Autodesk Inventor part; units mm, degrees
ref_plane "YZ Plane" through (0, 0, 0) normal (1, 0, 0) x (0, 1, 0)
ref_plane "XZ Plane" through (0, 0, 0) normal (0, 1, 0) x (-1, 0, 0)
ref_plane "XY Plane" through (0, 0, 0) normal (0, 0, 1) x (1, 0, 0)
sketch "Sketch1" plane through (0, 0, 0) normal (0, 0, 1) x (1, 0, 0)
  circle A0 centre (0, 0) radius 1.5875
  dimension "d0" = 3.175
extrude "Extrusion1" add sketch "Sketch1" along normal mid plane 33.0149
sketch "Sketch2" plane through (0, 0, 16.5075) normal (0, 0, 1) x (1, 0, 0)
  circle A0 centre (0, 0) radius 1.1913
  dimension "d3" = 2.3825
extrude "Extrusion2" add sketch "Sketch2" along normal blind 0.381
sketch "Sketch3" plane through (0, 0, 16.8885) normal (0, 0, 1) x (1, 0, 0)
  circle A0 centre (0, 0) radius 1.5875
  dimension "d6" = 3.175
extrude "Extrusion3" add sketch "Sketch3" along normal blind 1.27
chamfer "Chamfer1" distance 0.381 angle 45 1 edges at (-1.5875, 0, 18.1585)
mirror "Mirror1" about plane through (0, 0, 0) normal (0, 0, 1) of "Extrusion3", "Extrusion2", "Chamfer1"
scale "Scale1" factors (10, 10, 10) then translate (0, 0, 0) bodies 1
properties part number "Front Upper Hinge Pin"
Work out the finished part from the listing and answer in its coordinate system (mm). A direction names the side the tool comes from. Round coordinates to 2 decimals unless told otherwise and drop trailing zeros. Write each loop counter-clockwise with the first axis right and the second up, starting at its lowest first coordinate (ties: lowest second). Pieces come first, ordered by that corner, then holes. Notation, with made-up numbers: (57.25, 36.5) - (95.25, 36.5) arc R3 ccw to (95.25, 40.5) - close; hole circle Ø4 at (30, -18). An arc over 180 degrees is marked (long way). Answer in a Markdown table with one row per item. Add a question column.
1. The mould has two halves that part along Z. Classify faces 1 (the flat face through (2, 12, 165.074)), 2 (the flat face through (0, 0, -181.585)), 3 (the cylindrical face through (-3.441, -15.497, 2.311)): +Z half, -Z half, draft (parallel to the pull), parting line (faces both ways), or undercut.
2. For faces 4 (the flat face through (0, 0, 181.585)), 5 (the cylindrical face through (5.497, 10.569, 166.953)), determine the directions among +Z, -Z, +X, -X, +Y, -Y from which every point of the face is accessible in a straight line to the end or side of a thin tool.
3. Find the intervals of material crossed by line 1 along Z through (x, y) = (-13, 5) (1 decimal); line 2 along Z through (x, y) = (-5, 11.5) (1 decimal); line 3 along X through (y, z) = (-10.5, 4), in increasing order. Write a range as from..to.
4. Given pin 1 (3 mm diameter, centred on x = 8.5, z = 67.5, fed in from -Y); pin 2 (6 mm diameter, centred on y = 8, z = 23, fed in from +X); pin 3 (1.5 mm diameter, centred on y = -9, z = -81.5, fed in from +X), each flat-ended and moving along its own axis, determine where each tip first touches the part or whether it passes through.
5. A cutting plane is placed at A-A, the plane z = -25.5. Determine the outline of the cut face in (x, y) (3 decimals), and give its area (3 significant figures).
Worked out:
| question | item | result |
|---|---|---|
| 1 | face 1 | undercut |
| 1 | face 2 | -Z half |
| 1 | face 3 | draft |
| 2 | face 4 | +Z, +X, -X, +Y, -Y |
| 2 | face 5 | none |
| 3 | line 1 | -179.7..-168.9, -165.1..165.1, 168.9..179.7 |
| 3 | line 2 | -181.1..-168.9, -165.1..165.1, 168.9..181.1 |
| 3 | line 3 | -11.91..11.91 |
| 4 | pin 1 | y = -14.25 |
| 4 | pin 2 | x = 15.07 |
| 4 | pin 3 | x = 13.56 |
| 5 | outline | circle Ø31.75 at (0, 0) |
| 5 | area | 792 mm^2 |
